Geometry check sheet. Reference: the model listing, model coordinates, mm. Face numbers are marked on the shaded views. Round coordinates to 2 decimals unless told otherwise and drop trailing zeros. Order: outer loops, then holes, each group sorted by start corner. A loop starts at its lowest first (then second) coordinate and runs counter-clockwise, first axis right, second up. Notation, with made-up numbers: M 9,35.5 L 60,35.5 A34 ccw 60,68.5 Z; hole C 12,13 d7. An arc over 180 degrees is marked long. Answer as a JSON object with one key per item and string values. Group by question number.
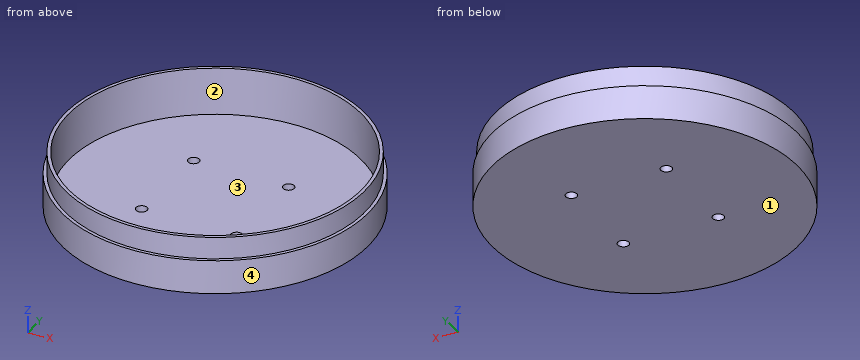
```python
from build123d import *

# Parameters (mm, degrees)
SKETCH1_R           = 44
SKETCH1_R_2         = 43
BOSS_EXTRUDE1_DEPTH = 14
SKETCH1_4_R         = 44
SKETCH1_4_R_2       = 43
BOSS_EXTRUDE2_DEPTH = 2.5
SKETCH5_W           = 1.65
SKETCH5_H           = 2.5
CIRPATTERN1_COUNT   = 4
SKETCH6_R           = 45
SKETCH6_R_2         = 44
BOSS_EXTRUDE3_DEPTH = 10


with BuildPart() as part:
    # Sketch1 → Boss-Extrude1 (new body)
    with BuildSketch(Plane.XY):
        Circle(SKETCH1_R)
        Circle(SKETCH1_R_2, mode=Mode.SUBTRACT)
    extrude(amount=BOSS_EXTRUDE1_DEPTH)



with BuildPart() as body_2:
    # Sketch1<4> → Boss-Extrude2 (new body)
    # profile 1 of 2: a face of its own
    with BuildSketch(Plane.XY):
        Circle(SKETCH1_4_R)
        Circle(SKETCH1_4_R_2, mode=Mode.SUBTRACT)
    # profile 2 of 2: a face of its own
    with BuildSketch(Plane.XY):
        Circle(SKETCH1_4_R_2)
    extrude(amount=-BOSS_EXTRUDE2_DEPTH)

    # Sketch5 → M4x0.7 Tapped Hole1 (revolve, cut)
    with BuildSketch(Plane(origin=(-14.142135624, 14.142135624, -2.5), x_dir=(0, 1, 0), z_dir=(1, 0, 0))):
        with Locations((0.825, 1.25)):
            Rectangle(SKETCH5_W, SKETCH5_H)
    m4x0_7_tapped_hole1 = revolve(axis=Axis((-14.142135624, 14.142135624, -8.85), (0, 0, 1)), mode=Mode.SUBTRACT)

    # CirPattern1: M4x0.7 Tapped Hole1 ×4 about axis
    cirpattern1_axis = Axis((0.019915384, -0.019915384, 0), (0, 0, 1))
    for i in range(1, CIRPATTERN1_COUNT):
        add(m4x0_7_tapped_hole1.rotate(cirpattern1_axis, i * 360 / CIRPATTERN1_COUNT), mode=Mode.SUBTRACT)


with BuildPart() as part_1:
    add(part.part)

    add(body_2.part)  # Boss-Extrude3 merges body 2
    # Sketch6 → Boss-Extrude3 (add)
    with BuildSketch(Plane(origin=(0, 0, -2.5), x_dir=(-1, 0, 0), z_dir=(0, 0, -1))):
        Circle(SKETCH6_R)
        Circle(SKETCH6_R_2, mode=Mode.SUBTRACT)
    extrude(amount=-BOSS_EXTRUDE3_DEPTH)


solid = part_1.part
```
1) Sectioned sample at D-D (z = 11.5). Record the boundary of the cut face in (x, y).
2) Sectioned sample at A-A (y = 0). Record the boundary of the cut face in (x, z).
3) Go/stop test with flat-tipped pins: P1, Ø2, axis at y = 31.5, z = 10, coming from the -X side; P2, Ø2, axis at x = 14.18, y = 14.14, coming from the +Z side; P3, Ø5, axis at x = 0.5, y = -26, coming from the +Z side; P4, Ø4, axis at x = 4.5, z = -1, coming from the -Y side. Record where each tip stops, or that it passes through.
4) Sectioned sample at B-B (z = 4.25). Record the boundary of the cut face in (x, y).
5) Thickness scan on line 1 along Z through (x, y) = (-5.5, 19); line 2 along X through (y, z) = (-20.5, 0.75); line 3 along Y through (x, z) = (0, 10.75). Record the ranges inside material, lowest first. Write a range as [from, to].
6) Release check for a two-part mould opening along Y. For the marked faces 1, 2, 3 and 4 record: +Y half, -Y half, draft (parallel to the pull), parting line (faces both ways), or undercut.
Final values:
{
 "1": {"outline": "C 0,0 d88; hole C 0,0 d86"},
 "2": {"outline": "M -45,-2.5 L 45,-2.5 L 45,7.5 L 44,7.5 L 44,14 L 43,14 L 43,0 L -43,0 L -43,14 L -44,14 L -44,7.5 L -45,7.5 Z"},
 "3": {"P1": "stops at x = -31.71", "P2": "passes through", "P3": "stops at z = 0", "P4": "stops at y = -44.93"},
 "4": {"outline": "C 0,0 d90; hole C 0,0 d86"},
 "5": {"line 1": "z = [-2.5, 0]", "line 2": "x = [-40.06, -37.8], [37.8, 40.06]", "line 3": "y = [-44, -43], [43, 44]"},
 "6": {"face 1": "draft", "face 2": "undercut", "face 3": "undercut", "face 4": "parting line"}
}
